from build123d import *

# Parameters (mm, degrees)
SKETCH_1_W          = 120
SKETCH_1_H          = 191
EXTRUDE_2_DEPTH     = 3
CHAMFER_7_SIZE      = 10
SKETCH_3_W          = 100
SKETCH_3_H          = 3
CUT_EXTRUDE_4_DEPTH = 1
SKETCH_6_W          = 3.195264444
SKETCH_6_H          = 39
CUT_EXTRUDE_5_DEPTH = 196.640080888
SKETCH_8_W          = 3
SKETCH_8_H          = 39
CUT_EXTRUDE_6_DEPTH = 196.640080888


with BuildPart() as part:
    # 草图1 → 凸台-拉伸2 (new body)
    with BuildSketch(Plane(origin=(0, 0, 0), x_dir=(1, 0, 0), z_dir=(0, 1, 0))):
        with Locations((15.482452441, -84.96728408)):
            Rectangle(SKETCH_1_W, SKETCH_1_H)
    extrude(amount=EXTRUDE_2_DEPTH)

    # 倒角7
    # the kernel refuses this chamfer: 10 mm, written as the material it takes off along each edge
    with BuildSketch(Plane(origin=(-44.517547559, 3, 206.18411396), x_dir=(-0.027495876610586317, -0.9996219169112968, 0), z_dir=(0, 0, -1))) as chamfer_7_piece_1:
        Polygon((CHAMFER_7_SIZE * 0.999621916911, -CHAMFER_7_SIZE * 0.0274958766106), (-CHAMFER_7_SIZE * 0.0274958766106, -CHAMFER_7_SIZE * 0.999621916911), (0, 0), align=None)
    extrude(amount=242.433659759, mode=Mode.SUBTRACT)

    # 草图3 → 切除-拉伸4 (cut)
    with BuildSketch(Plane(origin=(0, 3, 0), x_dir=(1, 0, 0), z_dir=(0, 1, 0))):
        with Locations((25.482452441, -178.96728408)):
            Rectangle(SKETCH_3_W, SKETCH_3_H)
        with Locations((25.482452441, 9.03271592)):
            Rectangle(SKETCH_3_W, SKETCH_3_H)
    extrude(amount=-CUT_EXTRUDE_4_DEPTH, mode=Mode.SUBTRACT)

    # 草图6 → 切除-拉伸5 (cut, through all)
    with BuildSketch(Plane(origin=(0, 0, 0), x_dir=(1, 0, 0), z_dir=(0, 1, 0))):
        with Locations((74.080084663, -11.96728408)):
            Rectangle(SKETCH_6_W, SKETCH_6_H)
    extrude(amount=CUT_EXTRUDE_5_DEPTH, mode=Mode.SUBTRACT)

    # 草图8 → 切除-拉伸6 (cut, through all)
    with BuildSketch(Plane(origin=(0, 0, 0), x_dir=(1, 0, 0), z_dir=(0, 1, 0))):
        with Locations((73.982452441, -157.96728408)):
            Rectangle(SKETCH_8_W, SKETCH_8_H)
    extrude(amount=CUT_EXTRUDE_6_DEPTH, mode=Mode.SUBTRACT)


solid = part.part
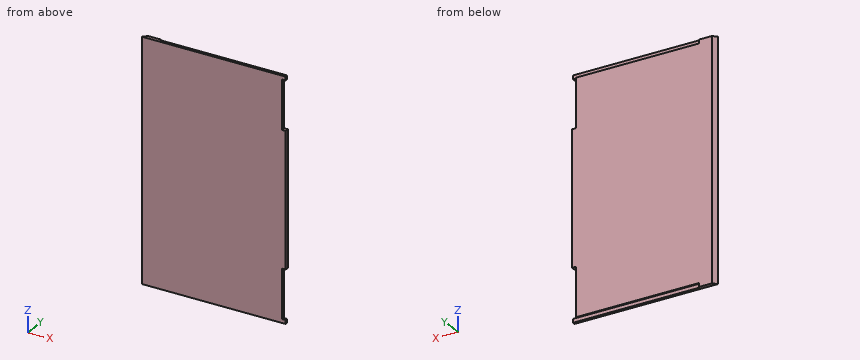
The listing builds one solid part. Answer for the finished solid, in the listing's coordinates (mm). Give positions to 0.01 mm unless a question says otherwise; leave off trailing zeros. Write each loop counter-clockwise with the first axis right and the second up, starting at its lowest first coordinate (ties: lowest second). Pieces come first, ordered by that corner, then holes. Notation, with made-up numbers: (-26.75, 71) - (19.25, 71) arc R28 cw to (19.25, 102) - close; hole circle Ø1 at (2.25, 34.25). An arc over 180 degrees is marked (long way). Use a Markdown table: item, result.
1. Section A-A on y = 0.9 is taken. Write down the section's boundary in (x, z).
Values follow:
| item | result |
|---|---|
| outline | (-36.62, -10.53) - (75.48, -10.53) - (75.48, -7.53) - (72.48, -7.53) - (72.48, 31.47) - (75.48, 31.47) - (75.48, 138.47) - (72.48, 138.47) - (72.48, 177.47) - (75.48, 177.47) - (75.48, 180.47) - (-36.62, 180.47) - close |
2. Find the intervals of material crossed by probe 1 along Z at (x, y) = (-21.5, 2.05); probe 2 along X at (y, z) = (2.75, 31.5); probe 3 along X at (y, z) = (1.7, 50), in increasing order. Write a range as from..to.
Values follow:
| item | result |
|---|---|
| probe 1 | z = -7.53..177.47 |
| probe 2 | x = -34.77..75.48 |
| probe 3 | x = -35.82..75.48 |
3. Section B-B on z = 147 is taken. Write down the section's boundary in (x, y), plus the area to 4 significant figures.
Values follow:
| item | result |
|---|---|
| outline | (-37.52, 0) - (72.48, 0) - (72.48, 3) - (-34.52, 3) - close |
| area | 325.5 mm² |
4. Each of these flat-tipped pins is pushed along its axis until it touches: P1, Ø0.9, axis at y = 1, z = 149, coming from the +X side; P2, Ø3.5, axis at x = 40, z = -9, coming from the +Y side; P3, Ø1.5, axis at x = 10.5, z = 179, coming from the +Y side; P4, Ø0.5, axis at y = 2.5, z = -8.5, coming from the +X side. Where does it stop, or does it pass through?
Values follow:
| item | result |
|---|---|
| P1 | stops at x = 72.48 |
| P2 | stops at y = 3 |
| P3 | stops at y = 2 |
| P4 | stops at x = -24.52 |
